```python
from build123d import *

# Parameters (mm, degrees)
F0_W     = 3
F0_H     = 3
F1_DEPTH = 4.65
F0_W_2   = 9.77
F0_H_2   = 8.07
F0_W_3   = 3.66
F2_DEPTH = 6.45
F0_R     = 1.25
F3_DEPTH = 0.44
F4_W     = 2
F4_H     = 0.55
F5_DEPTH = 3.88
F6_R     = 0.99999


# Not quite as in the source:
# - a fillet or chamfer is up to 0.001 mm smaller than in the source, because OpenCascade refuses the exact size


with BuildPart() as f1:
    # F0 (on Top) → F1 (new body)
    with BuildSketch(Plane.XY):
        with Locations((-1.83, 0)):
            Rectangle(F0_W, F0_H)
    extrude(amount=F1_DEPTH)

    # F0 (on Top) → F2 (join)
    with BuildSketch(Plane.XY):
        Rectangle(F0_W_2, F0_H_2)
        Polygon((-3.33, -1.5), (-3.33, 1.5), (-0.33, 1.5), (3.33, 1.5), (3.33, -1.5), (-0.33, -1.5), align=None, mode=Mode.SUBTRACT)
        with Locations((1.5, 0)):
            Rectangle(F0_W_3, F0_H)
        with Locations((-1.83, 0)):
            Rectangle(F0_W, F0_H)
    extrude(amount=-F2_DEPTH)

    # F0 (on Top) → F3 (join)
    with BuildSketch(Plane.XY):
        Polygon((-4.885, -4.035), (-4.885, 4.035), (-9.68, 2), (-9.68, -2), align=None)
        with Locations((-7.5463647954, 0)):
            Circle(F0_R, mode=Mode.SUBTRACT)
        Rectangle(F0_W_2, F0_H_2)
        Polygon((-3.33, -1.5), (-3.33, 1.5), (-0.33, 1.5), (3.33, 1.5), (3.33, -1.5), (-0.33, -1.5), align=None, mode=Mode.SUBTRACT)
        Polygon((9.68, 2), (4.885, 4.035), (4.885, -4.035), (9.68, -2), align=None)
        with Locations((7.5463647954, 0)):
            Circle(F0_R, mode=Mode.SUBTRACT)
    extrude(amount=F3_DEPTH)

    # F4 (on face) → F5 (join)
    with BuildSketch(Plane(origin=(0, 0, -6.45), x_dir=(1, 0, 0), z_dir=(0, 0, -1))):
        with Locations((-3.7156233341, 0)):
            Rectangle(F4_W, F4_H)
        with Locations((0.0545115434, 0)):
            Rectangle(F4_W, F4_H)
        with Locations((3.6328930184, 0)):
            Rectangle(F4_W, F4_H)
    extrude(amount=F5_DEPTH)

    # F6 (radius 1 in the source; OpenCascade refuses exactly that, so slightly less here)
    f6_edges = [f1.edges().sort_by_distance(p)[0] for p in [
        (-2.715623, 0, -10.33),
        (-4.715623, 0, -10.33),
        (-0.945488, 0, -10.33),
        (1.054512, 0, -10.33),
        (2.632893, 0, -10.33),
        (4.632893, 0, -10.33),
    ]]
    fillet(f6_edges, radius=F6_R)


solid = f1.part
```
The listing builds one solid part. Answer for the finished solid, in the listing's coordinates (mm). A direction names the side the tool comes from. Round coordinates to 2 decimals unless told otherwise and drop trailing zeros. Order: outer loops, then holes, each group sorted by start corner. A loop starts at its lowest first (then second) coordinate and runs counter-clockwise, first axis right, second up. Notation, with made-up numbers: (15, 3) - (25, 3) arc R20 cw to (25, 37) - close; hole circle Ø7 at (58.5, 7). An arc over 180 degrees is marked (long way). Put each result on its own line as item: value. Start each with the question number.
(1) Find section C-C (y = 1.75). Give the vertices of the cut face in (x, z) (3 decimals), plus the area to 3 significant figures.
(2) Given P1, Ø0.6, axis at x = 0, z = -8.5, coming from the -Y side (3 decimals); P2, Ø0.5, axis at x = 1.5, z = 0.5, coming from the +Y side (3 decimals); P3, Ø3, axis at y = -1, z = 3, coming from the -X side; P4, Ø3, axis at x = -6, y = 0, coming from the +Z side, each flat-ended and moving along its own axis, determine where each tip first touches the part or whether it passes through.
(3) Determine the mould class of faces 1 (the cylindrical face through (-8.795, 0.055, 0.217)), 2 (the cylindrical face through (0.77, 0, -10.03)), 3 (the flat face through (-2, 1.5, 3)) for opening direction Y: released by +Y, released by -Y, zero draft, split by the parting line, or undercut.
(4) Find section B-B (y = 0.5). Give the vertices of the cut face in (x, z) (3 decimals).
(5) Find section A-A (z = -8.75). Give the vertices of the cut face in (x, y) (3 decimals).
(6) For faces 4 (the flat face through (4.885, 0, -3)), 5 (the flat face through (-4.885, 0, -3)), 6 (the cylindrical face through (-3, 0, -10.03)), determine the directions among +Z, -Z, +X, -X, +Y, -Y from which every point of the face is accessible in a straight line to the end or side of a thin tool.
(7) Straight lines are drawn through the part: probe 1 along X at (y, z) = (0, -6.5); probe 2 along X at (y, z) = (1.25, 1.25); probe 3 along Z at (x, y) = (-3, 2.25). For each, find the intervals that lie inside material, in ascending order. Write a range as from..to.
(8) Find section D-D (x = -4.5). Give the vertices of the cut face in (y, z) (3 decimals).
Reply:
1. outline: (-9.68, 0) - (-4.885, 0) - (-4.885, -6.45) - (4.885, -6.45) - (4.885, 0) - (9.68, 0) - (9.68, 0.44) - (-9.68, 0.44) - close
1. area: 71.5 mm^2
2. P1: y = -0.275
2. P2: y = 4.035
2. P3: x = -3.33
2. P4: z = 0.44
3. face 1: undercut
3. face 2: zero draft
3. face 3: released by +Y
4. outline: (-9.68, 0) - (-8.692, 0) - (-8.692, 0.44) - (-9.68, 0.44) - close; (-6.401, 0) - (-4.885, 0) - (-4.885, -6.45) - (4.885, -6.45) - (4.885, 0) - (6.401, 0) - (6.401, 0.44) - (3.33, 0.44) - (3.33, 0) - (-0.33, 0) - (-0.33, 4.65) - (-3.33, 4.65) - (-3.33, 0.44) - (-6.401, 0.44) - close; (8.692, 0) - (9.68, 0) - (9.68, 0.44) - (8.692, 0.44) - close
5. outline: (-4.716, -0.275) - (-2.716, -0.275) - (-2.716, 0.275) - (-4.716, 0.275) - close; (-0.945, -0.275) - (1.055, -0.275) - (1.055, 0.275) - (-0.945, 0.275) - close; (2.633, -0.275) - (4.633, -0.275) - (4.633, 0.275) - (2.633, 0.275) - close
6. face 4: -Z, +X, +Y, -Y
6. face 5: -Z, -X, +Y, -Y
6. face 6: -Z, +Y, -Y
7. probe 1: -4.72..-2.72, -0.95..1.05, 2.63..4.63
7. probe 2: -3.33..-0.33
7. probe 3: -6.45..0.44
8. outline: (-4.035, -6.45) - (-0.275, -6.45) - (-0.275, -9.95) - (0.275, -9.95) - (0.275, -6.45) - (4.035, -6.45) - (4.035, 0.44) - (-4.035, 0.44) - close
